from build123d import *

# Parameters (mm, degrees)
F1_DEPTH = 8


with BuildPart() as f1:
    # F0 (on Front) → F1 (new body)
    with BuildSketch(Plane.XZ):
        with BuildLine():
            Line((0, 50.0126), (-6.0071, 50.0126))
            ThreePointArc((-6.0071, 50.0126), (-10.0076, 46.0121), (-14.0081, 50.0126))
            Line((-14.0081, 50.0126), (-20.0152, 50.0126))
            ThreePointArc((-20.0152, 50.0126), (-10.0076, 40.005), (0, 50.0126))
        make_face()
        with BuildLine():
            ThreePointArc((-14.0081, 50.0126), (-10.0076, 54.0131), (-6.0071, 50.0126))
            Line((-6.0071, 50.0126), (0, 50.0126))
            ThreePointArc((0, 50.0126), (-10.0076, 60.0202), (-20.0152, 50.0126))
            Line((-20.0152, 50.0126), (-14.0081, 50.0126))
        make_face()
        with BuildLine():
            Line((0, 0), (0, 50.0126))
            ThreePointArc((0, 50.0126), (-10.0076, 40.005), (-20.0152, 50.0126))
            Line((-20.0152, 50.0126), (-20.0152, 0))
            ThreePointArc((-20.0152, 0), (-10.0076, 10.0076), (0, 0))
        make_face()
        with BuildLine():
            ThreePointArc((-20.0152, 0), (-10.0076, -10.0076), (0, 0))
            Line((0, 0), (-6.0071, 0))
            ThreePointArc((-6.0071, 0), (-10.0076, -4.0005), (-14.0081, 0))
            Line((-14.0081, 0), (-20.0152, 0))
        make_face()
        with BuildLine():
            Line((-6.0071, 0), (0, 0))
            ThreePointArc((0, 0), (-10.0076, 10.0076), (-20.0152, 0))
            Line((-20.0152, 0), (-14.0081, 0))
            ThreePointArc((-14.0081, 0), (-10.0076, 4.0005), (-6.0071, 0))
        make_face()
    extrude(amount=F1_DEPTH)


solid = f1.part
Build history of the part. All positions in model axes, mm. Round coordinates to 2 decimals unless told otherwise and drop trailing zeros. Write each loop counter-clockwise with the first axis right and the second up, starting at its lowest first coordinate (ties: lowest second). Pieces come first, ordered by that corner, then holes. Notation, with made-up numbers: M -39.75,31.25 L -14.75,31.25 A32 cw -14.75,62.25 Z; hole C 66.5,-35.75 d6. An arc over 180 degrees is marked long. Answer as a JSON object with one key per item and string values. Group by question number.
(1) Cut at B-B (y = -4). Give the cut face in (x, z).
(2) Flat gauge pins, fed straight in: pin 1 (6 mm diameter, centred on x = -9, z = 47.5, fed in from +Y); pin 2 (1 mm diameter, centred on x = -18, y = -7, fed in from +Z); pin 3 (2 mm diameter, centred on x = -5, y = -6.5, fed in from +Z). Where does each tip first touch, or does it go through?
(3) Cut at A-A (x = -8). Give the cut face in (y, z).
(4) Cut at C-C (x = -19). Give the cut face in (y, z).
(5) Cut at D-D (x = -3.75). Give the cut face in (y, z), and give its area (3 significant figures).
(6) Mould opens along Z. For faces 1 (the cylindrical face through (-10.228, -3.944, -10.005)), 2 (the cylindrical face through (-6.19, -3.94, -1.2)), 3 (the flat face through (-20.015, -4, 25)) say: pulls with the +Z half, pulls with the -Z half, needs draft (parallel to the pull), parting line crosses it, or undercut.
(7) Drill centre lines: L1, parallel to Z at x = -11, y = -1.25; L2, parallel to Z at x = -11.75, y = -4.5; L3, parallel to X at y = -2, z = -2. Where is each one in solid material? Low to high.
Responses:
{
 "1": {"outline": "M -20.02,0 A10.01 ccw 0,0 L 0,50.01 A10.01 ccw -20.02,50.01 Z; hole C -10.01,0 d8; hole C -10.01,50.01 d8"},
 "2": {"pin 1": "stops at y = 0", "pin 2": "stops at z = 56.65", "pin 3": "stops at z = 59.18"},
 "3": {"outline": "M -8,-9.8 L 0,-9.8 L 0,-3.46 L -8,-3.46 Z; M -8,3.46 L 0,3.46 L 0,46.55 L -8,46.55 Z; M -8,53.47 L 0,53.47 L 0,59.82 L -8,59.82 Z"},
 "4": {"outline": "M -8,-4.39 L 0,-4.39 L 0,54.4 L -8,54.4 Z"},
 "5": {"outline": "M -8,-7.81 L 0,-7.81 L 0,57.82 L -8,57.82 Z", "area": "525 mm2"},
 "6": {"face 1": "pulls with the -Z half", "face 2": "undercut", "face 3": "needs draft"},
 "7": {"L1": "z = -9.96 to -3.88, 3.88 to 46.14, 53.89 to 59.97", "L2": "z = -9.85 to -3.6, 3.6 to 46.41, 53.61 to 59.87", "L3": "x = -19.81 to -13.47, -6.54 to -0.2"}
}
